```python
from build123d import *

# Parameters (mm, degrees)
F0_W     = 28
F0_H     = 25
F0_W_2   = 22.2
F0_H_2   = 19.2
F0_R     = 5
F1_DEPTH = 200
F2_DEPTH = 3
F3_W     = 22
F3_H     = 19
F4_DEPTH = 2.9


with BuildPart() as f1:
    # F0 (on Front) → F1 (new body)
    with BuildSketch(Plane.XZ):
        Rectangle(F0_W, F0_H)
        Rectangle(F0_W_2, F0_H_2, mode=Mode.SUBTRACT)
        Rectangle(F0_W_2, F0_H_2)
        Circle(F0_R, mode=Mode.SUBTRACT)
    extrude(amount=-F1_DEPTH)

    # F0 (on Front) → F2 (cut)
    with BuildSketch(Plane.XZ):
        Rectangle(F0_W_2, F0_H_2)
        Circle(F0_R, mode=Mode.SUBTRACT)
    extrude(amount=-F2_DEPTH, mode=Mode.SUBTRACT)

    # F3 (on face) → F4 (join)
    with BuildSketch(Plane(origin=(0, 200, 0), x_dir=(-1, 0, 0), z_dir=(0, 1, 0))):
        with Locations((0.121734367, 0.0437281778)):
            Rectangle(F3_W, F3_H)
        with BuildLine():
            ThreePointArc((-1.6292965707, 4.7270913557), (2.9717207978, 4.1519610515), (5.121734367, 0.0437281778))
            ThreePointArc((5.121734367, 0.0437281778), (4.1927589833, -2.8591597934), (1.7510309376, -4.6833631778))
            ThreePointArc((1.7510309376, -4.6833631778), (-4.7056209416, -1.690305166), (-1.6292965707, 4.7270913557))
        make_face(mode=Mode.SUBTRACT)
    extrude(amount=F4_DEPTH)


solid = f1.part
```
Geometry check sheet. Reference: the model listing, model coordinates, mm. Round coordinates to 2 decimals unless told otherwise and drop trailing zeros. Order: outer loops, then holes, each group sorted by start corner. A loop starts at its lowest first (then second) coordinate and runs counter-clockwise, first axis right, second up. Notation, with made-up numbers: (85.5, -34) -> (143.5, -34) arc R15 ccw to (143.5, -27) -> close; hole circle Ø10 at (-12, -3). An arc over 180 degrees is marked (long way). Return JSON: item names as keys, results as strings. Group by question number.
Q1. Material ranges on probe 1 along Z at (x, y) = (0, 70); probe 2 along X at (y, z) = (72, 0); probe 3 along Y at (x, z) = (-4, 6.75), recorded low to high. Write a range as from..to.
Q2. Section check A-A, the plane y = 141. Record the boundary of the cut face in (x, z), plus the area to 3 significant figures.
Q3. Gauge pin test, flat ends, axial feed: pin 1 (1.5 mm diameter, centred on x = -2, y = 202, fed in from -Z); pin 2 (8 mm diameter, centred on x = -5, z = 4.5, fed in from -Y); pin 3 (3 mm diameter, centred on y = 202, z = 0, fed in from -X); pin 4 (7.5 mm diameter, centred on x = 0, z = 0.5, fed in from +Y). Record the tip position at first contact, or that the pin passes through.
Q4. Release check for a two-part mould opening along Z. For faces 1 (the flat face through (0, 99, -12.5)), 2 (the flat face through (5, 202.9, 2)), 3 (the flat face through (0, 99, 12.5)), 4 (the flat face through (-5, 3, 2)) record: released by +Z, released by -Z, zero draft, split by the parting line, or undercut.
Numbers:
{
 "1": {"probe 1": "-12.5..-5, 5..12.5", "probe 2": "-14..-5, 5..14", "probe 3": "3..202.9"},
 "2": {"outline": "(-14, -12.5) -> (14, -12.5) -> (14, 12.5) -> (-14, 12.5) -> close; hole circle Ø10 at (0, 0)", "area": "621 mm^2"},
 "3": {"pin 1": "z = -9.46", "pin 2": "y = 3", "pin 3": "x = -11.12", "pin 4": "through"},
 "4": {"face 1": "released by -Z", "face 2": "zero draft", "face 3": "released by +Z", "face 4": "undercut"}
}
